Geometry check sheet. Reference: the model listing, model coordinates, mm. Face numbers are marked on the shaded views. Round coordinates to 2 decimals unless told otherwise and drop trailing zeros. Loops run counter-clockwise (first coordinate to the right, second up) from the corner with the lowest first, then second, coordinate; pieces in that order, holes last. Notation, with made-up numbers: (40.25, 14.5) -> (71.25, 14.5) arc R5 ccw to (71.25, 23.5) -> close; hole circle Ø3 at (-5, 45.5). An arc over 180 degrees is marked (long way). Use a Markdown table: item, result. Add a question column.
Q1. Sectioned sample at C-C, the plane z = 2. Enter the section's corners in (x, y), then the cut area to 4 significant figures.
Q2. Release check for a two-part mould opening along Y. For the marked faces 1, 2, 3 and 4 record: released by +Y, released by -Y, zero draft, split by the parting line, or undercut.
Q3. Gauge pin test, flat ends, axial feed: P1, Ø1.2, axis at x = 63, y = 5.5, coming from the +Z side; P2, Ø1, axis at x = 65.5, y = 9, coming from the +Z side; P3, Ø6, axis at x = 21, y = 8, coming from the +Z side. Record the tip position at first contact, or that the pin passes through.
Q4. Sectioned sample at A-A, the plane y = 46.5. Enter the section's corners in (x, z).
Q5. Material ranges on L1, parallel to Y at x = 24, z = 5.5; L2, parallel to Y at x = 6, z = 7.25; L3, parallel to Z at x = 76.5, y = 40.5, recorded low to high.
Q6. Sectioned sample at B-B, the plane x = 55. Enter the section's corners in (y, z), then the cut area to 4 significant figures.
Q7. Sectioned sample at D-D, the plane z = 7. Give the number of separate pieces and of enclosed holes in the cut face, then the cut area to 3 significant figures.
```python
from build123d import *

# Parameters (mm, degrees)
F0_W      = 89
F0_H      = 60
F1_DEPTH  = 1
F2_W      = 89
F2_H      = 60
F2_W_2    = 86
F2_H_2    = 57
F3_DEPTH  = 10.5
F4_W      = 15
F4_H      = 11.5
F5_DEPTH  = 1.5
F6_W      = 10
F6_H      = 7.5
F6_W_2    = 18
F6_H_2    = 6.5
F6_W_3    = 8.5
F7_DEPTH  = 1.5
F8_W      = 17.5
F8_H      = 8.5
F8_W_2    = 16
F9_DEPTH  = 1.5
F10_R     = 1.25
F11_DEPTH = 9
F12_W     = 8
F12_H     = 8
F12_R     = 1.25
F13_DEPTH = 2


with BuildPart() as f1:
    # F0 (on Top) → F1 (new body)
    with BuildSketch(Plane.XY):
        with Locations((44.5, 30)):
            Rectangle(F0_W, F0_H)
    extrude(amount=F1_DEPTH)

    # F2 (on face) → F3 (join)
    with BuildSketch(Plane.XY.offset(1)):
        with Locations((44.5, 30)):
            Rectangle(F2_W, F2_H)
        with Locations((44.5, 30)):
            Rectangle(F2_W_2, F2_H_2, mode=Mode.SUBTRACT)
    extrude(amount=F3_DEPTH)

    # F4 (on face) → F5 (cut, through all)
    with BuildSketch(Plane(origin=(0, 0, 0), x_dir=(0, -1, 0), z_dir=(-1, 0, 0))):
        with Locations((-30, 5.75)):
            Rectangle(F4_W, F4_H)
    extrude(amount=-F5_DEPTH, mode=Mode.SUBTRACT)

    # F6 (on face) → F7 (cut, through all)
    with BuildSketch(Plane.XZ):
        with Locations((12.5, 7.75)):
            Rectangle(F6_W, F6_H)
        with Locations((34, 8.25)):
            Rectangle(F6_W_2, F6_H_2)
        with Locations((55.5, 7.75)):
            Rectangle(F6_W_3, F6_H)
    extrude(amount=-F7_DEPTH, mode=Mode.SUBTRACT)

    # F8 (on face) → F9 (cut, through all)
    with BuildSketch(Plane.YZ.offset(89)):
        with Locations((11.75, 7.25)):
            Rectangle(F8_W, F8_H)
        with Locations((30.5, 7.25)):
            Rectangle(F8_W_2, F8_H)
        with Locations((48.5, 7.25)):
            Rectangle(F8_W_2, F8_H)
    extrude(amount=-F9_DEPTH, mode=Mode.SUBTRACT)

    # F10 (on face) → F11 (join)
    with BuildSketch(Plane.XY.offset(1)):
        with Locations((5.5, 54.5)):
            Circle(F10_R)
        with Locations((63.5, 54.5)):
            Circle(F10_R)
        with Locations((5.5, 5.5)):
            Circle(F10_R)
        with Locations((63.5, 5.5)):
            Circle(F10_R)
    extrude(amount=F11_DEPTH)

    # F12 (on face) → F13 (join)
    with BuildSketch(Plane.XY.offset(1)):
        with Locations((5.5, 54.5)):
            Rectangle(F12_W, F12_H)
        with Locations((5.5, 54.5)):
            Circle(F12_R, mode=Mode.SUBTRACT)
        with Locations((63.5, 54.5)):
            Rectangle(F12_W, F12_H)
        with Locations((63.5, 54.5)):
            Circle(F12_R, mode=Mode.SUBTRACT)
        with Locations((63.5, 5.5)):
            Rectangle(F12_W, F12_H)
        with Locations((63.5, 5.5)):
            Circle(F12_R, mode=Mode.SUBTRACT)
        with Locations((5.5, 5.5)):
            Rectangle(F12_W, F12_H)
        with Locations((5.5, 5.5)):
            Circle(F12_R, mode=Mode.SUBTRACT)
    extrude(amount=F13_DEPTH)


solid = f1.part
```
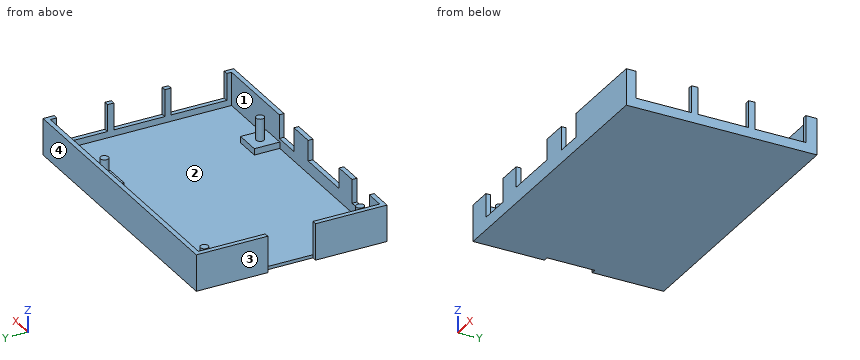
Values:
| question | item | result |
|---|---|---|
| 1 | outline | (0, 0) -> (89, 0) -> (89, 60) -> (0, 60) -> (0, 37.5) -> (1.5, 37.5) -> (1.5, 50.5) -> (9.5, 50.5) -> (9.5, 58.5) -> (59.5, 58.5) -> (59.5, 50.5) -> (67.5, 50.5) -> (67.5, 58.5) -> (87.5, 58.5) -> (87.5, 1.5) -> (67.5, 1.5) -> (67.5, 9.5) -> (59.5, 9.5) -> (59.5, 1.5) -> (9.5, 1.5) -> (9.5, 9.5) -> (1.5, 9.5) -> (1.5, 22.5) -> (0, 22.5) -> close |
| 1 | area | 671.5 mm^2 |
| 2 | face 1 | undercut |
| 2 | face 2 | undercut |
| 2 | face 3 | zero draft |
| 2 | face 4 | released by +Y |
| 3 | P1 | z = 10 |
| 3 | P2 | z = 3 |
| 3 | P3 | z = 1 |
| 4 | outline | (0, 0) -> (89, 0) -> (89, 3) -> (87.5, 3) -> (87.5, 1) -> (1.5, 1) -> (1.5, 11.5) -> (0, 11.5) -> close |
| 5 | L1 | 0 to 1.5, 58.5 to 60 |
| 5 | L2 | 0 to 1.5, 4.35 to 6.65, 53.35 to 55.65, 58.5 to 60 |
| 5 | L3 | 0 to 1 |
| 6 | outline | (0, 0) -> (60, 0) -> (60, 11.5) -> (58.5, 11.5) -> (58.5, 1) -> (1.5, 1) -> (1.5, 4) -> (0, 4) -> close |
| 6 | area | 80.25 mm^2 |
| 7 | separate pieces | 11 |
| 7 | enclosed holes | 0 |
| 7 | area | 306 mm^2 |
